Autodesk Inventor part; units mm, degrees
ref_plane "YZ Plane" through (0, 0, 0) normal (1, 0, 0) x (0, 1, 0)
ref_plane "XZ Plane" through (0, 0, 0) normal (0, 1, 0) x (-1, 0, 0)
ref_plane "XY Plane" through (0, 0, 0) normal (0, 0, 1) x (1, 0, 0)
sketch "스케치1" plane through (0, 0, 0) normal (1, 0, 0) x (0, 1, 0)
  line L0 (0, 0) -> (0, 58.2)
  line L1 (0, 58.2) -> (18.65, 58.2)
  line L2 (0, 0) -> (37.3, 0)
  circle A0 centre (37.3, 7.4) radius 7.4
  circle A1 centre (37.3, 7.4) radius 3
  line L3 (18.65, 58.2) -> (43.8327, 10.8763)
  dimension "d3" = 14.8
  dimension "d0" = 58.2
  dimension "d1" = 37.3
  dimension "d2" = 18.65
  dimension "d4" = 0
  dimension "d5" = 6
extrude "돌출1" add sketch "스케치1" along normal mid plane 26.2
sketch "스케치2" plane through (-13.1, 0, 58.2) normal (0, 0, 1) x (1, 0, 0)
  line L0 (3, 3) -> (23.2, 3)
  line L1 (23.2, 3) -> (23.2, 55.8283)
  line L2 (23.2, 55.8283) -> (3, 55.8283)
  line L3 (3, 55.8283) -> (3, 3)
  line L4 (26.2, 43.8327) -> (26.2, 18.65)
  line L5 (26.2, 0) -> (0, 0)
  line L6 (0, 18.65) -> (0, 43.8327)
  point P0 (13.1, 0)
  dimension "d8" = 3
  dimension "d9" = 3
  dimension "d10" = 3
extrude "돌출2" cut sketch "스케치2" against normal through all
sketch "스케치3" plane through (-10.1, 3, 58.2) normal (0, 1, 0) x (1, 0, 0)
  circle A0 centre (10.1, 48.6) radius 4.5
  line L0 (0, 58.2) -> (20.2, 58.2)
  line L1 (14.6, 58.2) -> (5.6, 58.2)
  line L2 (5.6, 58.2) -> (5.6, 48.6)
  line L3 (5.6, 48.6) -> (14.6, 48.6)
  line L4 (14.6, 48.6) -> (14.6, 58.2)
  circle A1 centre (10.1, 12.3112) radius 4.25
  point P0 (10.1, 58.2)
  point P1 (10.1, 58.2)
  point P2 (10.1, 48.6)
  point P3 (10.1, 58.2)
  point P4 (14.6, 48.6)
  dimension "d13" = 9
  dimension "d14" = 9
  dimension "d15" = 9.6
  dimension "d16" = 0
  dimension "d17" = 8.5
  dimension "d18" = 0
extrude "돌출3" cut sketch "스케치3" against normal through all
equation "\"d2\" = 0.5 * d1"
properties part number "높이액추브라켓"
The listing builds one solid part. Answer for the finished solid, in the listing's coordinates (mm). A direction names the side the tool comes from. Round coordinates to 2 decimals unless told otherwise and drop trailing zeros. Loops run counter-clockwise (first coordinate to the right, second up) from the corner with the lowest first, then second, coordinate; pieces in that order, holes last. Notation, with made-up numbers: (74, 52.25) - (111, 52.25) arc R11 cw to (111, 56.25) - close; hole circle Ø5 at (54, 11). An arc over 180 degrees is marked (long way). Return JSON: item names as keys, results as strings. Group by question number.
1. The part is cut by section A-A on z = 7.4. Determine the outline of the cut face in (x, y), then the cut area to 3 significant figures.
2. This flat-tipped pin is pushed along its axis until it touches: P1, Ø10, axis at x = -3.5, z = 15.5, coming from the +Y side. Where does it stop, or does it pass through?
3. Which of the six approach directions +Z, -Z, +X, -X, +Y, -Y give full straight-line access (tool end or side, diameter ignored) to faces 5 (the flat face through (10.1, 19, 23)), 6 (the flat face through (-11.621, 31.065, 34.869)), 7 (the flat face through (4.5, 2, 5))?
4. The part is cut by section B-B on y = 10. Determine the outline of the cut face in (x, z).
5. The part is cut by section C-C on x = 0. Determine the outline of the cut face in (y, z), then the cut area to 3 significant figures.
6. Consider probe 1 along Z at (x, y) = (0, 0.75); probe 2 along Y at (x, z) = (11.05, 7.4); probe 3 along X at (y, z) = (11, 53.5). Determine where each line is inside the solid, lowest interval first.
7. The mould has two halves that part along X. Classify faces 1 (the flat face through (-4.5, 2, 5)), 2 (the cylindrical face through (11.579, 43.698, 3.682)), 3 (the flat face through (0, 3, 30)), 4 (the flat face through (13.1, 17, 23)): pulls with the +X half, pulls with the -X half, needs draft (parallel to the pull), parting line crosses it, or undercut.
8. The part is cut by section D-D on z = 15. Determine the outline of the cut face in (x, y), then the cut area to 3 significant figures.
Resolved:
{
 "1": {"outline": "(-13.1, 0) - (-4.5, 0) - (-4.5, 3) - (-10.1, 3) - (-10.1, 34.3) - (-13.1, 34.3) - close; (-13.1, 40.3) - (-10.1, 40.3) - (-10.1, 44.7) - (-13.1, 44.7) - close; (4.5, 0) - (13.1, 0) - (13.1, 34.3) - (10.1, 34.3) - (10.1, 3) - (4.5, 3) - close; (10.1, 40.3) - (13.1, 40.3) - (13.1, 44.7) - (10.1, 44.7) - close", "area": "266 mm²"},
 "2": {"P1": "stops at y = 3"},
 "3": {"face 5": "+Z, -Z, +Y", "face 6": "+Z, +X, -X, +Y", "face 7": "-Z, +Y, -Y"},
 "4": {"outline": "(-13.1, 0) - (-10.1, 0) - (-10.1, 58.2) - (-13.1, 58.2) - close; (10.1, 0) - (13.1, 0) - (13.1, 58.2) - (10.1, 58.2) - close"},
 "5": {"outline": "(0, 14.1) - (3, 14.1) - (3, 41.64) - (0, 41.64) - close; (0, 50.14) - (3, 50.14) - (3, 58.2) - (0, 58.2) - close", "area": "107 mm²"},
 "6": {"probe 1": "z = 14.1 to 41.64, 50.14 to 58.2", "probe 2": "y = 0 to 34.3, 40.3 to 44.7", "probe 3": "x = -13.1 to -10.1, 10.1 to 13.1"},
 "7": {"face 1": "undercut", "face 2": "needs draft", "face 3": "undercut", "face 4": "pulls with the +X half"},
 "8": {"outline": "(-13.1, 0) - (13.1, 0) - (13.1, 41.64) - (10.1, 41.64) - (10.1, 3) - (-10.1, 3) - (-10.1, 41.64) - (-13.1, 41.64) - close", "area": "310 mm²"}
}
